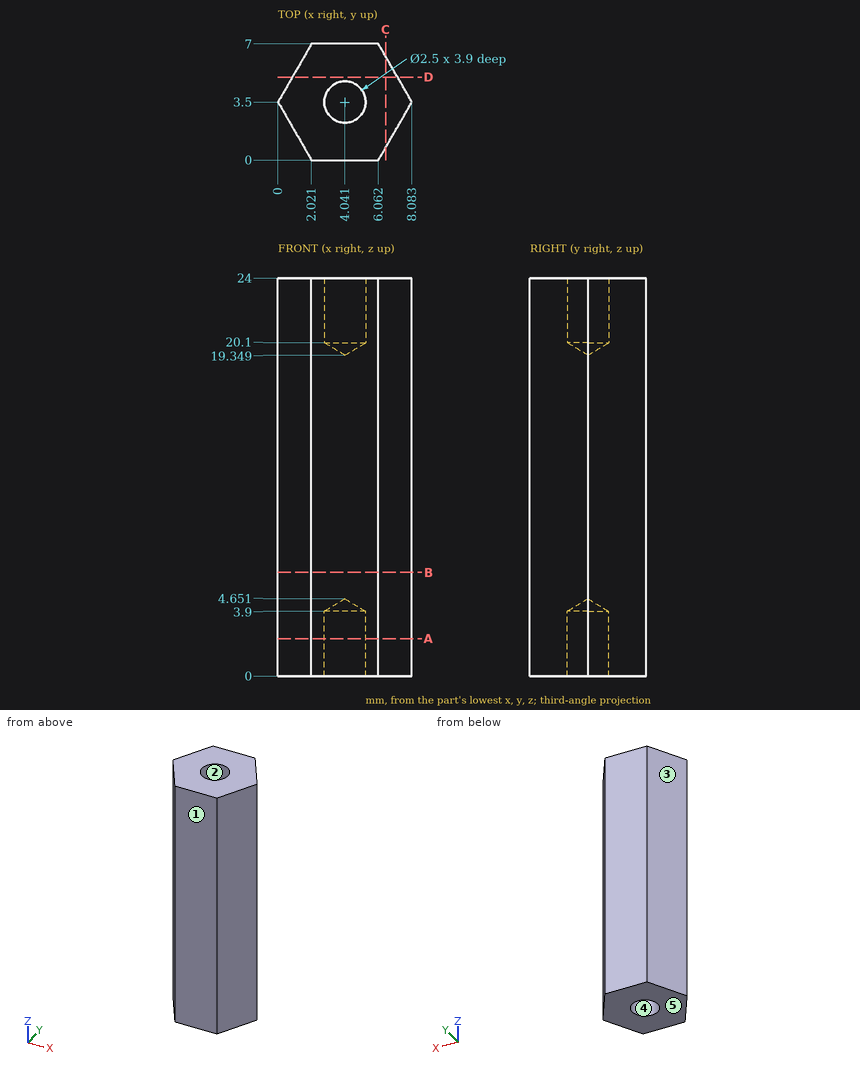
Part print with two shaded views. Sizes in mm from the minimum x, y, z corner. A direction names the side the tool comes from. Coordinates: 2 decimals unless noted, no trailing zeros. Write each loop counter-clockwise with the first axis right and the second up, starting at its lowest first coordinate (ties: lowest second). Pieces come first, ordered by that corner, then holes.
1. 3-axis set-ups, long thin cutter, end or side, ignore diameter. For the marked faces 4 and 5: which of +Z, -Z, +X, -X, +Y, -Y reach the whole face in a straight line?
Answer block:
face 4: -Z
face 5: -Z, +X, -X, +Y, -Y
2. Pull direction Y, two halves, no side cores. Call the marked faces 1, 2 and 3: released by +Y, released by -Y, zero draft, split by the parting line, or undercut.
Answer block:
face 1: released by -Y
face 2: undercut
face 3: released by +Y
3. Drill centre lines: probe 1 along Y at (x, z) = (6.5, 8) (1 decimal); probe 2 along X at (y, z) = (5, 13) (1 decimal); probe 3 along X at (y, z) = (3.75, 13.75) (1 decimal). Where is each one in solid material? Low to high.
Answer block:
probe 1: y = 0.8 to 6.2
probe 2: x = 0.9 to 7.2
probe 3: x = 0.1 to 7.9
4. Band-saw the part on B-B, the plane z = 6.25. Give the cut face in (x, y).
Answer block:
outline: (0, 3.5) - (2.02, 0) - (6.06, 0) - (8.08, 3.5) - (6.06, 7) - (2.02, 7) - close
5. Band-saw the part on D-D, the plane y = 5. Give the cut face in (x, z), and give its area (3 significant figures).
Answer block:
outline: (0.87, 0) - (7.22, 0) - (7.22, 24) - (0.87, 24) - close
area: 152 mm2
6. Band-saw the part on A-A, the plane z = 2.25. Give the cut face in (x, y).
Answer block:
outline: (0, 3.5) - (2.02, 0) - (6.06, 0) - (8.08, 3.5) - (6.06, 7) - (2.02, 7) - close; hole circle Ø2.5 at (4.04, 3.5)
7. Drop flat-ended pins along their axis: pin 1 (1.5 mm diameter, centred on x = 7, y = 1.5, fed in from +Z); pin 2 (3 mm diameter, centred on y = 5.5, z = 4.5, fed in from +X) (1 decimal). Give the stop position or say it passes through.
Answer block:
pin 1: stops at z = 24
pin 2: stops at x = 7.8
8. Band-saw the part on C-C, the plane x = 6.5. Give the cut face in (y, z), and give its area (3 significant figures).
Answer block:
outline: (0.76, 0) - (6.24, 0) - (6.24, 24) - (0.76, 24) - close
area: 132 mm2
